The model under review builds one solid part; all positions refer to its coordinate system, in mm. A direction names the side the tool comes from. Coordinates: 2 decimals unless noted, no trailing zeros. Write each loop counter-clockwise with the first axis right and the second up, starting at its lowest first coordinate (ties: lowest second). Pieces come first, ordered by that corner, then holes. Notation, with made-up numbers: (54.5, 39) -> (89.5, 39) arc R18 ccw to (89.5, 56) -> close; hole circle Ø1 at (-33, 40.5). An arc over 180 degrees is marked (long way). Write each question's results on one line, items separated by ' | '.
Autodesk Fusion 360 part; units mm, degrees
sketch "Sketch1" plane through (0, 0, 0) normal (0, 0, 1) x (1, 0, 0)
  line L0 (15, -15) -> (-15, -15)
  line L1 (-15, -15) -> (-15, 15)
  line L2 (-10, 15) -> (-10, 27)
  line L3 (-10, 27) -> (10, 27)
  line L4 (10, 27) -> (10, 15)
  line L5 (-5, 19) -> (-5, 23)
  line L6 (-5, 23) -> (5, 23)
  line L7 (5, 23) -> (5, 19)
  line L8 (-15, 15) -> (-10, 15)
  line L9 (10, 15) -> (15, 15)
  line L10 (0, 70) -> (0, -30) construction
  line L11 (15, 0.5) -> (12, 0.5)
  line L12 (12, 4.5) -> (15, 4.5)
  arc A0 (12, 4.5) -> (12, 0.5) centre (12, 2.5) ccw
  line L13 (15, 15) -> (15, 4.5)
  line L14 (15, 0.5) -> (15, -15)
  circle A1 centre (2, 11.25) radius 1.5
  circle A2 centre (2, -6.25) radius 1.5
  line L15 (-5, 19) -> (5, 19)
  dimension "d1" = 30
  dimension "d3" = 12
  dimension "d4" = 20
  dimension "d7" = 4
  dimension "d8" = 10
  dimension "d9" = 42
  dimension "d17" = 12.5
  dimension "d18" = 2
  dimension "d21" = 17.5
  dimension "d22" = 3
  dimension "d23" = 3
  dimension "d24" = 10
  dimension "d25" = 3
  dimension "d29" = 4
extrude "Extrude1" add sketch "Sketch1" along normal blind 4
Q1. Machinability: for faces 1 (the flat face through (5, 21, 2)), 2 (the flat face through (-13, 15, 2)), 3 (the flat face through (14, 0.5, 2)), which of the approach directions +Z, -Z, +X, -X, +Y, -Y give a long, thin tool a straight path to every point of the face, cutting with its end or side? Answer none if there is none.
Solution:
face 1: +Z, -Z | face 2: +Z, -Z, -X, +Y | face 3: +Z, -Z, +X
Q2. Add section A-A (x = 2). Write out the cut boundary in (y, z), plus the area to 3 significant figures.
Solution:
outline: (-15, 0) -> (-7.75, 0) -> (-7.75, 4) -> (-15, 4) -> close; (-4.75, 0) -> (9.75, 0) -> (9.75, 4) -> (-4.75, 4) -> close; (12.75, 0) -> (19, 0) -> (19, 4) -> (12.75, 4) -> close; (23, 0) -> (27, 0) -> (27, 4) -> (23, 4) -> close | area: 128 mm²
Q3. Add section C-C (z = 3.4). Write out the cut boundary in (x, y), plus the area to 3 significant figures.
Solution:
outline: (-15, -15) -> (15, -15) -> (15, 0.5) -> (12, 0.5) arc R2 cw to (12, 4.5) -> (15, 4.5) -> (15, 15) -> (10, 15) -> (10, 27) -> (-10, 27) -> (-10, 15) -> (-15, 15) -> close; hole (-5, 19) -> (5, 19) -> (5, 23) -> (-5, 23) -> close; hole circle Ø3 at (2, -6.25); hole circle Ø3 at (2, 11.25) | area: 1,070 mm²
Q4. Add section D-D (x = 13.25). Write out the cut boundary in (y, z).
Solution:
outline: (-15, 0) -> (0.5, 0) -> (0.5, 4) -> (-15, 4) -> close; (4.5, 0) -> (15, 0) -> (15, 4) -> (4.5, 4) -> close
Q5. For line 1 (Y direction, x = 2, z = 2.75); line 2 (Y direction, x = -1, z = 3.8); line 3 (X direction, y = 22, z = 0.5), list the stretches that pass through material, from the lowest coordinate up. Write a range as from..to.
Solution:
line 1: -15..-7.75, -4.75..9.75, 12.75..19, 23..27 | line 2: -15..19, 23..27 | line 3: -10..-5, 5..10
Q6. Clearance check with flat-ended pins moving along their axes: P1, Ø1.2, axis at x = -12.5, z = 1.5, coming from the +Y side; P2, Ø1.8, axis at x = 2, y = -6.25, coming from the +Z side. State where each tip first meets the part, or that it passes through.
Solution:
P1: y = 15 | P2: through
Q7. Add section B-B (y = 11.25). Write out the cut boundary in (x, z).
Solution:
outline: (-15, 0) -> (0.5, 0) -> (0.5, 4) -> (-15, 4) -> close; (3.5, 0) -> (15, 0) -> (15, 4) -> (3.5, 4) -> close
Q8. Draft analysis for pull direction X (two halves, no side actions). For faces 4 (the flat face through (12, 15, 2)), 5 (the cylindrical face through (1.675, 12.714, 1.972)), 6 (the flat face through (-15, 0, 2)), state which applies: pulls with the +X half, pulls with the -X half, needs draft (parallel to the pull), parting line crosses it, or undercut.
Solution:
face 4: needs draft | face 5: undercut | face 6: pulls with the -X half
